from build123d import *

# Parameters (mm, degrees)
SKETCH1_W           = 40
SKETCH1_H           = 17
BOSS_EXTRUDE1_DEPTH = 1.4
CUT_EXTRUDE1_START  = 1.4
SKETCH3_W           = 16
SKETCH3_H           = 4
SKETCH3_W_2         = 3
SKETCH3_H_2         = 11
CUT_EXTRUDE1_DEPTH  = 1
SKETCH4_R           = 1.3
CUT_EXTRUDE2_DEPTH  = 11
SKETCH7_W           = 9
SKETCH7_H           = 17
CUT_EXTRUDE5_DEPTH  = 21
SKETCH9_W           = 16
SKETCH9_H           = 20.041444064
SKETCH9_R           = 2.55
BOSS_EXTRUDE3_DEPTH = 3
FILLET1_R           = 10


with BuildPart() as part:
    # Sketch1 → Boss-Extrude1 (new body)
    with BuildSketch(Plane.XY):
        Rectangle(SKETCH1_W, SKETCH1_H)
    extrude(amount=BOSS_EXTRUDE1_DEPTH)

    # Sketch3 → Cut-Extrude1 (cut)
    with BuildSketch(Plane.XY.offset(CUT_EXTRUDE1_START)):
        with Locations((7, -1)):
            Rectangle(SKETCH3_W, SKETCH3_H)
        with Locations((-9.5, -1)):
            Rectangle(SKETCH3_W_2, SKETCH3_H_2)
    extrude(amount=-CUT_EXTRUDE1_DEPTH, mode=Mode.SUBTRACT)

    # Sketch4 → Cut-Extrude2 (cut)
    with BuildSketch(Plane.XY):
        with Locations(Location((16, 5, 0), (0, 0, 180))):
            Circle(SKETCH4_R)
        with Locations(Location((-3, 5, 0), (0, 0, 180))):
            Circle(SKETCH4_R)
    extrude(amount=CUT_EXTRUDE2_DEPTH, mode=Mode.SUBTRACT)

    # Sketch7 → Cut-Extrude5 (cut)
    with BuildSketch(Plane.XY):
        with Locations((-15.5, 0)):
            Rectangle(SKETCH7_W, SKETCH7_H)
    extrude(amount=CUT_EXTRUDE5_DEPTH, mode=Mode.SUBTRACT)

    # Sketch9 → Boss-Extrude3 (add)
    with BuildSketch(Plane.XY):
        with Locations((15, -18.520722032)):
            Rectangle(SKETCH9_W, SKETCH9_H)
        with Locations((15, -13)):
            Circle(SKETCH9_R, mode=Mode.SUBTRACT)
        with Locations((15, -24)):
            Circle(SKETCH9_R, mode=Mode.SUBTRACT)
    extrude(amount=BOSS_EXTRUDE3_DEPTH)

    # Fillet1
    # the kernel refuses this fillet: 10 mm, written as the material it adds along each edge
    with BuildSketch(Plane(origin=(7, -8.5, 0), x_dir=(-1, 0, 0), z_dir=(0, 0, 1))) as fillet1_piece_1:
        with BuildLine():
            CenterArc((FILLET1_R, FILLET1_R), FILLET1_R, 180, 90)
            Line((0, FILLET1_R), (0, 0))
            Line((0, 0), (FILLET1_R, 0))
        make_face()
    extrude(amount=1.4)
    with BuildSketch(Plane(origin=(20, -8.5, 0), x_dir=(0, 1, 0), z_dir=(0, 0, 1))) as fillet1_piece_2:
        with BuildLine():
            CenterArc((7.141428429, -10), FILLET1_R, 90, 45.572995999)
            Line((0, -3), (0, 0))
            Line((0, 0), (7.141428429, 0))
        make_face()
    extrude(amount=1.4)


solid = part.part
Can you work these out from the model? Positions are in its coordinate system, mm. A direction names the side the tool comes from. Give positions to 0.01 mm unless a question says otherwise; leave off trailing zeros. Loops run counter-clockwise (first coordinate to the right, second up) from the corner with the lowest first, then second, coordinate; pieces in that order, holes last. Notation, with made-up numbers: (74.25, -26.75) -> (102.25, -26.75) arc R17 ccw to (102.25, 4.25) -> close; hole circle Ø2 at (50, 86). An arc over 180 degrees is marked (long way). Write item = value, one per line.
1) Suppose I cut it at C-C on y = 5. Write out the boundary of the cut face in (x, z).
Check result:
outline = (-11, 0) -> (-4.3, 0) -> (-4.3, 1.4) -> (-11, 1.4) -> close; (-1.7, 0) -> (14.7, 0) -> (14.7, 1.4) -> (-1.7, 1.4) -> close; (17.3, 0) -> (20, 0) -> (20, 1.4) -> (17.3, 1.4) -> close
2) Suppose I cut it at D-D on x = 16. Write out the boundary of the cut face in (y, z).
Check result:
outline = (-28.54, 0) -> (-26.35, 0) -> (-26.35, 3) -> (-28.54, 3) -> close; (-21.65, 0) -> (-15.35, 0) -> (-15.35, 3) -> (-21.65, 3) -> close; (-10.65, 0) -> (3.7, 0) -> (3.7, 1.4) -> (-8.5, 1.4) -> (-8.5, 3) -> (-10.65, 3) -> close; (6.3, 0) -> (8.5, 0) -> (8.5, 1.4) -> (6.3, 1.4) -> close
3) I need wall thicknesses on L1, parallel to X at y = 5, z = 0.6; L2, parallel to Y at x = -3, z = 0.6; L3, parallel to Y at x = 16, z = 1.05. Which ranges of each line are inside material? Lowest first, please. Write a range as from..to.
Check result:
L1 = -11..-4.3, -1.7..14.7, 17.3..20
L2 = -8.5..3.7, 6.3..8.5
L3 = -28.54..-26.35, -21.65..-15.35, -10.65..3.7, 6.3..8.5
4) Thinking about a two-plate mould opening in X: for faces 5 (the flat face through (-10, -1, 0.4)), 6 (the cylindrical face through (17.03, 5.79, 0.69)), 7 (the flat face through (23, -19, 1)), 8 (the flat face through (7, -21, 2)), which applies, released by +X, released by -X, zero draft, split by the parting line, or undercut?
Check result:
face_5 = zero draft
face_6 = undercut
face_7 = released by +X
face_8 = released by -X
5) Suppose I cut it at A-A on y = -24. Write out the boundary of the cut face in (x, z), then the cut area to 3 significant figures.
Check result:
outline = (7, 0) -> (12.45, 0) -> (12.45, 3) -> (7, 3) -> close; (17.55, 0) -> (23, 0) -> (23, 3) -> (17.55, 3) -> close
area = 32.7 mm2
6) Will these pins go through, and if not, where does the flat tip stop? pin 1 (1.5 mm diameter, centred on x = -8.5, z = 0.5, fed in from -Y); pin 2 (1.5 mm diameter, centred on y = 2.5, z = 0.5, fed in from +X); pin 3 (3 mm diameter, centred on x = 9, y = 0, fed in from +Z); pin 4 (6 mm diameter, centred on x = 15, y = -24, fed in from -Z).
Check result:
pin_1 = -8.5
pin_2 = 20
pin_3 = 1.4
pin_4 = 0
7) For faces 1 (the flat face through (20, 4, 1)), 2 (the flat face through (-7, -8.5, 1)), 3 (the flat face through (7, -1, 0.4)), 4 (the flat face through (15, -8.5, 2)), which set-ups out of +Z, -Z, +X, -X, +Y, -Y let a thin tool reach every point of the face, with its end or its side?
Check result:
face_1 = +Z, -Z, +X, +Y
face_2 = +Z, -Z, -X, -Y
face_3 = +Z
face_4 = +Z, +X, -X, +Y
8) Suppose I cut it at B-B on z = 1.95. Write out the boundary of the cut face in (x, y).
Check result:
outline = (7, -28.54) -> (23, -28.54) -> (23, -8.5) -> (7, -8.5) -> close; hole circle Ø5.1 at (15, -24); hole circle Ø5.1 at (15, -13)
